from build123d import *

# Parameters (mm, degrees)
F0_R     = 15
F1_DEPTH = 20.32
F2_DEPTH = 20.32


with BuildPart() as f1:
    # F0 (on Top) → F1 (new body)
    with BuildSketch(Plane.XY):
        Circle(F0_R)
        with BuildLine():
            ThreePointArc((1.863643, 1.666384), (2.335499, 0.891878), (2.5, 0))
            ThreePointArc((2.5, 0), (1.767767, -1.767767), (0, -2.5))
            ThreePointArc((0, -2.5), (-2.2821, -1.020794), (-1.863643, 1.666384))
            ThreePointArc((-1.863643, 1.666384), (0, 2.5), (1.863643, 1.666384))
        make_face(mode=Mode.SUBTRACT)
    extrude(amount=F1_DEPTH)

    # F0 (on Top) → F2 (join)
    with BuildSketch(Plane.XY):
        with BuildLine():
            Line((0, 1.666384), (1.863643, 1.666384))
            ThreePointArc((1.863643, 1.666384), (0, 2.5), (-1.863643, 1.666384))
            Line((-1.863643, 1.666384), (0, 1.666384))
        make_face()
    extrude(amount=F2_DEPTH)


solid = f1.part
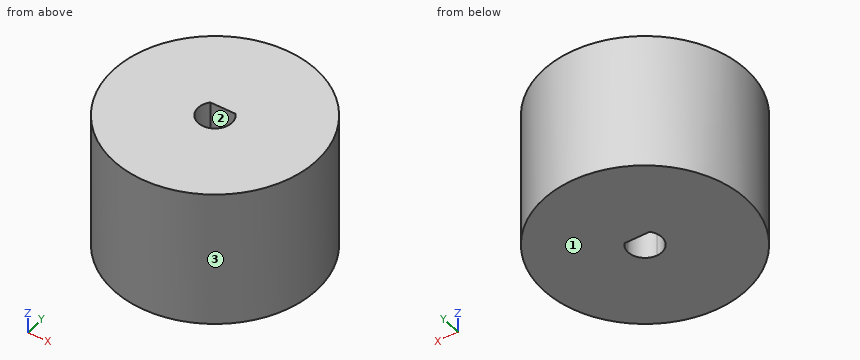
Here's how the part is built. I have some questions about the finished solid (model axes, mm). Face numbers are marked on the shaded views. Coordinates: 2 decimals unless noted, no trailing zeros. Loops run counter-clockwise (first coordinate to the right, second up) from the corner with the lowest first, then second, coordinate; pieces in that order, holes last.
1. Imagine slicing it at D-D, the plane x = 11.5. Please give me the cut outline in (y, z).
2. If we mould it in two halves opening along Y, with no side actions, what happens to the marked faces 1, 2 and 3? For each: pulls with the +Y half, pulls with the -Y half, needs draft (parallel to the pull), parting line crosses it, or undercut.
3. Imagine slicing it at A-A, the plane y = -0.75. Please give me the cut outline in (x, z).
4. Imagine slicing it at C-C, the plane z = 6. Please give me the cut outline in (x, y).
5. For P1, Ø8, axis at y = 3.5, z = 9, coming from the -X side; P2, Ø3, axis at y = 3, z = 16.5, coming from the -X side; P3, Ø1, axis at x = -7, z = 10, coming from the +Y side; P4, Ø4, axis at x = 2.5, z = 12.5, coming from the +Y side, each with a flat end and sliding along its axis, tell me the tip position at first contact or that it passes through.
6. I need wall thicknesses on L1, parallel to Y at x = 2.25, z = 14; L2, parallel to Y at x = 1.25, z = 11.75; L3, parallel to Y at x = -4.5, z = 7. Which ranges of each line are inside material? Lowest first, please.
7. Imagine slicing it at B-B, the plane x = -1. Please give me the cut outline in (y, z), and give its area (3 significant figures).
Taken from the geometry:
1. outline: (-9.63, 0) - (9.63, 0) - (9.63, 20.32) - (-9.63, 20.32) - close
2. face 1: needs draft
2. face 2: undercut
2. face 3: parting line crosses it
3. outline: (-14.98, 0) - (-2.38, 0) - (-2.38, 20.32) - (-14.98, 20.32) - close; (2.38, 0) - (14.98, 0) - (14.98, 20.32) - (2.38, 20.32) - close
4. outline: circle Ø30 at (0, 0); hole (-1.86, 1.67) arc R2.5 ccw (long way) to (2.5, 0) arc R2.5 ccw to (1.86, 1.67) - close
5. P1: stops at x = -15
5. P2: stops at x = -14.92
5. P3: stops at y = 13.52
5. P4: stops at y = 14.99
6. L1: y = -14.83 to -1.09, 1.09 to 14.83
6. L2: y = -14.95 to -2.17, 1.67 to 14.95
6. L3: y = -14.31 to 14.31
7. outline: (-14.97, 0) - (-2.29, 0) - (-2.29, 20.32) - (-14.97, 20.32) - close; (1.67, 0) - (14.97, 0) - (14.97, 20.32) - (1.67, 20.32) - close
7. area: 528 mm2
